The model under review builds one solid part; all positions refer to its coordinate system, in mm. A direction names the side the tool comes from. Coordinates: 2 decimals unless noted, no trailing zeros. Write each loop counter-clockwise with the first axis right and the second up, starting at its lowest first coordinate (ties: lowest second). Pieces come first, ordered by that corner, then holes. Notation, with made-up numbers: (56.25, -12) - (64.25, -12) arc R29 cw to (64.25, 26) - close; hole circle Ø11 at (-3.5, 14). An arc over 180 degrees is marked (long way). Return JSON: item names as keys, results as strings. Group by question number.
(1) Draft analysis for pull direction Y (two halves, no side actions). For faces 1 (the face through (267.33, 0.29, 1.96)), 2 (the face through (-4, 15.875, 2)), 3 (the face through (1, 14, 139.7)), state which applies: released by +Y, released by -Y, zero draft, split by the parting line, or undercut.
(2) We need section C-C on z = 10. State the section outline as (x, y) points (3 decimals).
(3) Tool access review of faces 4 (the face through (-4, 13.335, 2)), 5 (the face through (-269.87, -0.35, 1.96)): name each direction out of +Z, -Z, +X, -X, +Y, -Y from which nothing blocks a thin tool from reaching the whole face with its end or side.
(4) We need section B-B on y = 0. State the section outline as (x, z) points (3 decimals), then the cut area to 3 significant figures.
(5) For pin 1 Ø3 at (y, z) = (-7, -54) entering from +X, flat-tipped, find the tip position at first contact; note if it passes through.
(6) We need section A-A on x = 29. State the section outline as (y, z) points (3 decimals).
(7) To check wall thickness, follow L1, parallel to Y at x = -3.5, z = 108 (3 decimals); L2, parallel to X at y = 0.5, z = 51; L3, parallel to X at y = 1, z = -89. State the ranges of each line that lie inside material, in increasing order. Write a range as from..to.
```python
from build123d import *

# Parameters (mm, degrees)
BOSS_EXTRU_1_DEPTH      = 139.7
ENL_V_MAT_EXTRU_1_REACH = 390.779


with BuildPart() as part:
    # Esquisse1 → Boss.-Extru.1 (new, symmetric)
    with BuildSketch(Plane.XY):
        with BuildLine():
            Line((-254, 15.875), (254, 15.875))
            ThreePointArc((254, 15.875), (269.875, 0), (254, -15.875))
            Line((254, -15.875), (-254, -15.875))
            ThreePointArc((-254, -15.875), (-269.875, 0), (-254, 15.875))
        make_face()
    extrude(amount=BOSS_EXTRU_1_DEPTH, both=True)

    # Esquisse2 → Enlèv. mat.-Extru.1 (cut, up to next)
    with BuildSketch(Plane.XY.offset(139.7), mode=Mode.PRIVATE) as enl_v_mat_extru_1_sk1:
        with BuildLine():
            Line((-254, 13.335), (254, 13.335))
            ThreePointArc((254, 13.335), (267.335, 0), (254, -13.335))
            Line((254, -13.335), (-254, -13.335))
            ThreePointArc((-254, -13.335), (-267.335, 0), (-254, 13.335))
        make_face()
    enl_v_mat_extru_1_tool1 = extrude(enl_v_mat_extru_1_sk1.sketch, amount=-ENL_V_MAT_EXTRU_1_REACH, mode=Mode.PRIVATE) & part.part
    add(enl_v_mat_extru_1_tool1.solids().sort_by_distance((0, 0, 139.7))[0], mode=Mode.SUBTRACT)


solid = part.part
```
Ans:
{
 "1": {"face 1": "undercut", "face 2": "released by +Y", "face 3": "zero draft"},
 "2": {"outline": "(-254, -15.875) - (254, -15.875) arc R15.875 ccw to (254, 15.875) - (-254, 15.875) arc R15.875 ccw to start; hole (-254, -13.335) - (254, -13.335) arc R13.335 ccw to (254, 13.335) - (-254, 13.335) arc R13.335 ccw to start"},
 "3": {"face 4": "+Z, -Z", "face 5": "+Z, -Z, -X"},
 "4": {"outline": "(-269.875, -139.7) - (-267.335, -139.7) - (-267.335, 139.7) - (-269.875, 139.7) - close; (267.335, -139.7) - (269.875, -139.7) - (269.875, 139.7) - (267.335, 139.7) - close", "area": "1,420 mm²"},
 "5": {"pin 1": "x = 268.89"},
 "6": {"outline": "(-15.875, -139.7) - (-13.335, -139.7) - (-13.335, 139.7) - (-15.875, 139.7) - close; (13.335, -139.7) - (15.875, -139.7) - (15.875, 139.7) - (13.335, 139.7) - close"},
 "7": {"L1": "-15.875..-13.335, 13.335..15.875", "L2": "-269.87..-267.33, 267.33..269.87", "L3": "-269.84..-267.3, 267.3..269.84"}
}
